from build123d import *

# Parameters (mm, degrees)
BOSS_EXTRUDE1_DEPTH = 16.637
SKETCH2_R           = 4.1656
CUT_EXTRUDE1_DEPTH  = 77.2
SKETCH3_R           = 4.1656
CUT_EXTRUDE2_DEPTH  = 77.2


with BuildPart() as part:
    # Sketch1 → Boss-Extrude1 (new body, symmetric)
    with BuildSketch(Plane.XY):
        with BuildLine():
            Line((0, 0), (0, 76.2))
            ThreePointArc((0, 76.2), (4.490128061, 74.340128061), (6.35, 69.85))
            Line((6.35, 69.85), (6.35, 14.2748))
            ThreePointArc((6.35, 14.2748), (8.67112018, 8.67112018), (14.2748, 6.35))
            Line((14.2748, 6.35), (69.85, 6.35))
            ThreePointArc((69.85, 6.35), (74.340128061, 4.490128061), (76.2, 0))
            Line((76.2, 0), (0, 0))
        make_face()
    extrude(amount=BOSS_EXTRUDE1_DEPTH, both=True)

    # Sketch2 → Cut-Extrude1 (cut, through all)
    with BuildSketch(Plane(origin=(0, 0, 0), x_dir=(1, 0, 0), z_dir=(0, 1, 0))):
        with Locations((19.05, 0)):
            Circle(SKETCH2_R)
        with Locations((57.15, 0)):
            Circle(SKETCH2_R)
    extrude(amount=CUT_EXTRUDE1_DEPTH, mode=Mode.SUBTRACT)

    # Sketch3 → Cut-Extrude2 (cut, through all)
    with BuildSketch(Plane(origin=(0, 0, 0), x_dir=(0, 0, -1), z_dir=(1, 0, 0))):
        with Locations((0, 19.05)):
            Circle(SKETCH3_R)
        with Locations((0, 57.15)):
            Circle(SKETCH3_R)
    extrude(amount=CUT_EXTRUDE2_DEPTH, mode=Mode.SUBTRACT)


solid = part.part
The listing builds one solid part. Answer for the finished solid, in the listing's coordinates (mm). A direction names the side the tool comes from. Round coordinates to 2 decimals unless told otherwise and drop trailing zeros. Order: outer loops, then holes, each group sorted by start corner. A loop starts at its lowest first (then second) coordinate and runs counter-clockwise, first axis right, second up. Notation, with made-up numbers: (-39, -24.75) - (-7, -24.75) arc R16 ccw to (-7, -12.75) - close; hole circle Ø5 at (-8, 84.25). An arc over 180 degrees is marked (long way). Write item = value, one per line. Start each with the question number.
1) Section A-A, the plane y = 19.05 is taken. Write down the section's boundary in (x, z).
2) Section D-D, the plane z = 10 is taken. Write down the section's boundary in (x, y), plus the area to 3 significant figures.
3) For a pull along Z with two mould halves and no side action, classify faces 3 (the cylindrical face through (23.023, 3.131, -1.251)), 4 (the flat face through (21, 4, 16.637)), 5 (the cylindrical face through (4.44, 74.39, 0.23)) as released by +Z, released by -Z, zero draft, split by the parting line, or undercut.
4) Given pin 1 (4 mm diameter, centred on y = 40.5, z = 13, fed in from +X); pin 2 (6 mm diameter, centred on x = 38.5, z = 12, fed in from +Y), each flat-ended and moving along its own axis, determine where each tip first touches the part or whether it passes through.
5) Straight lines are drawn through the part: L1, parallel to Z at x = 2.5, y = 19.05; L2, parallel to X at y = 5, z = 0; L3, parallel to Y at x = 2.25, z = 0. For each, find the intervals that lie inside material, in ascending order.
6) For faces 1 (the cylindrical face through (52.99, 3.13, -0.18)), 2 (the flat face through (6.35, 42, 0)), determine the directions among +Z, -Z, +X, -X, +Y, -Y from which every point of the face is accessible in a straight line to the end or side of a thin tool.
7) Section C-C, the plane z = 0 is taken. Write down the section's boundary in (x, y), plus the area to 3 significant figures.
Results list:
q1.outline = (0, -16.64) - (6.35, -16.64) - (6.35, -4.17) - (0, -4.17) - close; (0, 4.17) - (6.35, 4.17) - (6.35, 16.64) - (0, 16.64) - close
q2.outline = (0, 0) - (76.2, 0) arc R6.35 ccw to (69.85, 6.35) - (14.27, 6.35) arc R7.92 cw to (6.35, 14.27) - (6.35, 69.85) arc R6.35 ccw to (0, 76.2) - close
q2.area = 924 mm^2
q3.face_3 = undercut
q3.face_4 = released by +Z
q3.face_5 = zero draft
q4.pin_1 = 6.35
q4.pin_2 = 6.35
q5.L1 = -16.64 to -4.17, 4.17 to 16.64
q5.L2 = 0 to 14.88, 23.22 to 52.98, 61.32 to 73.76
q5.L3 = 0 to 14.88, 23.22 to 52.98, 61.32 to 75.79
q6.face_1 = +Y, -Y
q6.face_2 = +Z, -Z, +X, +Y
q7.outline = (0, 0) - (14.88, 0) - (14.88, 6.35) - (14.27, 6.35) arc R7.92 cw to (6.35, 14.27) - (6.35, 14.88) - (0, 14.88) - close; (0, 23.22) - (6.35, 23.22) - (6.35, 52.98) - (0, 52.98) - close; (0, 61.32) - (6.35, 61.32) - (6.35, 69.85) arc R6.35 ccw to (0, 76.2) - close; (23.22, 0) - (52.98, 0) - (52.98, 6.35) - (23.22, 6.35) - close; (61.32, 0) - (76.2, 0) arc R6.35 ccw to (69.85, 6.35) - (61.32, 6.35) - close
q7.area = 712 mm^2
